Solid Edge part; units mm, degrees
sketch "Sketch1" plane through (0, 0, 0) normal (0, 0, 1) x (1, 0, 0)
  line L0 (-94.5, 46) -> (-85.5, 46)
  line L1 (-85.5, 46) -> (-85.5, 55.5)
  line L2 (-85.5, 55.5) -> (-94.5, 55.5)
  line L3 (-94.5, 55.5) -> (-94.5, 46)
  line L4 (-94.5, 4) -> (-85.5, 4)
  line L5 (-85.5, -5.5) -> (-85.5, 4)
  line L6 (-94.5, -5.5) -> (-85.5, -5.5)
  line L7 (-94.5, 4) -> (-94.5, -5.5)
  line L8 (-52.5, 4) -> (-43.5, 4)
  line L9 (-43.5, -5.5) -> (-43.5, 4)
  line L10 (-52.5, -5.5) -> (-43.5, -5.5)
  line L11 (-52.5, 4) -> (-52.5, -5.5)
  line L12 (-52.5, 46) -> (-43.5, 46)
  line L13 (-43.5, 46) -> (-43.5, 55.5)
  line L14 (-43.5, 55.5) -> (-52.5, 55.5)
  line L15 (-52.5, 55.5) -> (-52.5, 46)
extrude "Protrusion1" add sketch "Sketch1" along normal blind 4
sketch "Sketch2" plane through (-97, -4.7, 4) normal (0, 0, 1) x (1, 0, 0)
  line L0 (-4.7, 52.4) -> (60.7, 52.4)
  line L1 (60.7, 52.4) -> (60.7, 7)
  line L2 (60.7, 7) -> (-4.7, 7)
  line L3 (-4.7, 7) -> (-4.7, 52.4)
extrude "ExtrudedProtrusion_2" add sketch "Sketch2" against normal blind 2.2
sketch "Sketch3" plane through (-61.5, 21.5, 1.8) normal (0, 0, -1) x (0, -1, 0)
  line L0 (17.5, -21.7) -> (17.5, -23.5)
  line L1 (17.5, -23.5) -> (-24.5, -23.5)
  line L2 (-24.5, -23.5) -> (-24.5, 38.5)
  line L3 (-24.5, 38.5) -> (17.5, 38.5)
  line L4 (17.5, 38.5) -> (17.5, 36.7)
  line L5 (17.5, 36.7) -> (17.5, 20.3)
  line L6 (17.5, 20.3) -> (17.5, -5.3)
  line L7 (17.5, -5.3) -> (17.5, -21.7)
extrude "ExtrudedCutout_1" cut sketch "Sketch3" against normal blind 1
hole "Hole_1" at (-90, 51, 4) direction (0, 0, -1) diameter 3.6 end up to next counterbore diameter 7 counterbore depth 2.5
hole "Hole1" at (-48, 51, 4) direction (0, 0, -1) diameter 3.6 end up to next counterbore diameter 7 counterbore depth 2.5
hole "Hole2" at (-48, -1, 4) direction (0, 0, -1) diameter 3.6 end up to next counterbore diameter 7 counterbore depth 2.5
hole "Hole3" at (-90, -1, 4) direction (0, 0, -1) diameter 3.6 end up to next counterbore diameter 7 counterbore depth 2.5
fillet "Round_1" radius 1 16 edges at (-36.3, 2.3, 2.9) (-36.3, 47.7, 2.9) (-101.7, 2.3, 2.9) (-101.7, 47.7, 2.9) (-43.5, -5.5, 2) (-52.5, -5.5, 2) (-94.5, -5.5, 2) (-85.5, -5.5, 2) (-85.5, 55.5, 2) (-94.5, 55.5, 2) (-52.5, 55.5, 2) (-43.5, 55.5, 2) (-38, 4, 2.3) (-100, 4, 2.3) (-38, 46, 2.3) (-100, 46, 2.3)
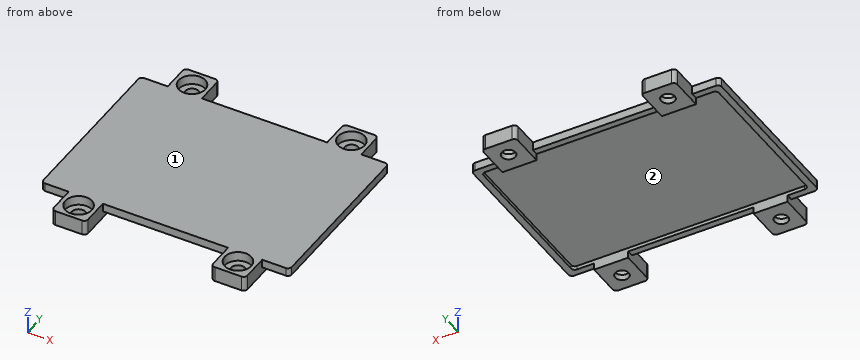
The listing builds one solid part. Answer for the finished solid, in the listing's coordinates (mm). Face numbers are marked on the shaded views. Give positions to 0.01 mm unless a question says otherwise; leave off trailing zeros. Order: outer loops, then holes, each group sorted by start corner. A loop starts at its lowest first (then second) coordinate and runs counter-clockwise, first axis right, second up.
Item 1: The part is cut by section A-A, the plane z = 0.9. Give the vertices of the cut face in (x, y), and give its area (3 significant figures).
From the geometry:
outline: (-94.5, -4.5) arc R1 ccw to (-93.5, -5.5) - (-86.5, -5.5) arc R1 ccw to (-85.5, -4.5) - (-85.5, 4) - (-94.5, 4) - close; (-94.5, 46) - (-85.5, 46) - (-85.5, 54.5) arc R1 ccw to (-86.5, 55.5) - (-93.5, 55.5) arc R1 ccw to (-94.5, 54.5) - close; (-52.5, -4.5) arc R1 ccw to (-51.5, -5.5) - (-44.5, -5.5) arc R1 ccw to (-43.5, -4.5) - (-43.5, 4) - (-52.5, 4) - close; (-52.5, 46) - (-43.5, 46) - (-43.5, 54.5) arc R1 ccw to (-44.5, 55.5) - (-51.5, 55.5) arc R1 ccw to (-52.5, 54.5) - close; hole circle Ø3.6 at (-90, -1); hole circle Ø3.6 at (-90, 51); hole circle Ø3.6 at (-48, -1); hole circle Ø3.6 at (-48, 51)
area: 300 mm2
Item 2: Given pin 1 Ø1 at (x, z) = (-56.5, 3.5) entering from -Y; pin 2 Ø0.9 at (x, y) = (-62.5, 46.5) entering from -Z; pin 3 Ø2 at (x, y) = (-48, -1) entering from -Z; pin 4 Ø6 at (x, y) = (-70.5, 11.5) entering from -Z, each flat-ended and moving along its own axis, determine where each tip first touches the part or whether it passes through.
From the geometry:
pin 1: stops at y = 2.3
pin 2: stops at z = 1.8
pin 3: passes through
pin 4: stops at z = 2.8
Item 3: The part is cut by section D-D, the plane y = 15. Give the vertices of the cut face in (x, z).
From the geometry:
outline: (-101.7, 1.8) - (-100, 1.8) - (-100, 2.8) - (-38, 2.8) - (-38, 1.8) - (-36.3, 1.8) - (-36.3, 4) - (-101.7, 4) - close
Item 4: The part is cut by section B-B, the plane y = 51. Give the vertices of the cut face in (x, z).
From the geometry:
outline: (-94.5, 0) - (-91.8, 0) - (-91.8, 1.5) - (-93.5, 1.5) - (-93.5, 4) - (-94.5, 4) - close; (-88.2, 0) - (-85.5, 0) - (-85.5, 4) - (-86.5, 4) - (-86.5, 1.5) - (-88.2, 1.5) - close; (-52.5, 0) - (-49.8, 0) - (-49.8, 1.5) - (-51.5, 1.5) - (-51.5, 4) - (-52.5, 4) - close; (-46.2, 0) - (-43.5, 0) - (-43.5, 4) - (-44.5, 4) - (-44.5, 1.5) - (-46.2, 1.5) - close
Item 5: For a pull along Y with two mould halves and no side action, classify the marked faces 1 and 2 as pulls with the +Y half, pulls with the -Y half, needs draft (parallel to the pull), parting line crosses it, or undercut.
From the geometry:
face 1: needs draft
face 2: undercut
Item 6: The part is cut by section C-C, the plane x = -90. Give the vertices of the cut face in (y, z).
From the geometry:
outline: (-5.5, 0) - (-2.8, 0) - (-2.8, 1.5) - (-4.5, 1.5) - (-4.5, 4) - (-5.5, 4) - close; (0.8, 0) - (4, 0) - (4, 2.8) - (46, 2.8) - (46, 0) - (49.2, 0) - (49.2, 1.5) - (47.5, 1.5) - (47.5, 4) - (2.5, 4) - (2.5, 1.5) - (0.8, 1.5) - close; (52.8, 0) - (55.5, 0) - (55.5, 4) - (54.5, 4) - (54.5, 1.5) - (52.8, 1.5) - close
Item 7: Find the intervals of material crossed by probe 1 along X at (y, z) = (51, 2.1); probe 2 along X at (y, z) = (51, 1.1); probe 3 along Y at (x, z) = (-90, 0.4), in increasing order.
From the geometry:
probe 1: x = -94.5 to -93.5, -86.5 to -85.5, -52.5 to -51.5, -44.5 to -43.5
probe 2: x = -94.5 to -91.8, -88.2 to -85.5, -52.5 to -49.8, -46.2 to -43.5
probe 3: y = -5.5 to -2.8, 0.8 to 4, 46 to 49.2, 52.8 to 55.5
